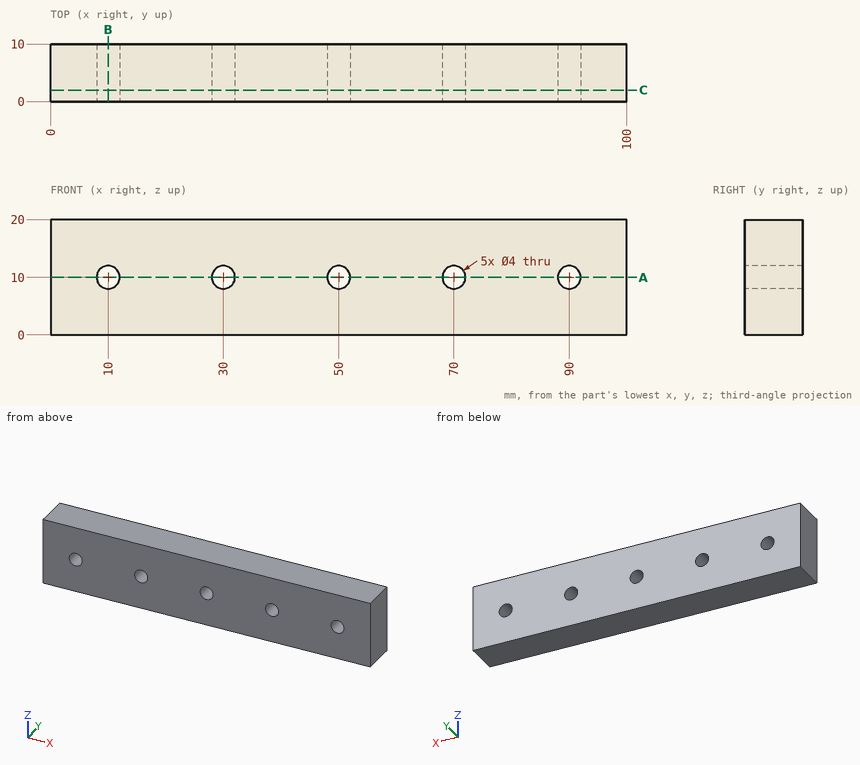
The drawing under review shows one solid part. Ordinate dimensions are in mm from its lowest x, y, z. Round coordinates to 2 decimals unless told otherwise and drop trailing zeros. Loops run counter-clockwise (first coordinate to the right, second up) from the corner with the lowest first, then second, coordinate; pieces in that order, holes last. Notation, with made-up numbers: (74, 9.5) - (129, 9.5) arc R22 cw to (129, 34.5) - close; hole circle Ø4 at (88, 21.5). An arc over 180 degrees is marked (long way). One line per item, written item: value. Start each with the question number.
1) To check wall thickness, follow L1, parallel to X at y = 2.5, z = 10; L2, parallel to Z at x = 30, y = 4.5; L3, parallel to X at y = 9.75, z = 8.5. State the ranges of each line that lie inside material, in increasing order. Write a range as from..to.
2) Insertion check: pin 1 Ø2.5 at (x, z) = (50, 10) entering from +Y; pin 2 Ø4.5 at (x, z) = (90, 10) entering from -Y. Each pin has a flat end and moves straight along its axis. Give the tip position at first contact, or say it passes through.
3) Consider section A-A on z = 10. Give the boundary of the cut face in (x, y), then the cut area to 3 significant figures.
4) Consider section C-C on y = 2. Give the boundary of the cut face in (x, z).
5) Consider section B-B on x = 10. Give the boundary of the cut face in (y, z), then the cut area to 3 significant figures.
Reported:
1. L1: x = 0..8, 12..28, 32..48, 52..68, 72..88, 92..100
1. L2: z = 0..8, 12..20
1. L3: x = 0..8.68, 11.32..28.68, 31.32..48.68, 51.32..68.68, 71.32..88.68, 91.32..100
2. pin 1: passes through
2. pin 2: stops at y = 0
3. outline: (0, 0) - (8, 0) - (8, 10) - (0, 10) - close; (12, 0) - (28, 0) - (28, 10) - (12, 10) - close; (32, 0) - (48, 0) - (48, 10) - (32, 10) - close; (52, 0) - (68, 0) - (68, 10) - (52, 10) - close; (72, 0) - (88, 0) - (88, 10) - (72, 10) - close; (92, 0) - (100, 0) - (100, 10) - (92, 10) - close
3. area: 800 mm^2
4. outline: (0, 0) - (100, 0) - (100, 20) - (0, 20) - close; hole circle Ø4 at (10, 10); hole circle Ø4 at (30, 10); hole circle Ø4 at (50, 10); hole circle Ø4 at (70, 10); hole circle Ø4 at (90, 10)
5. outline: (0, 0) - (10, 0) - (10, 8) - (0, 8) - close; (0, 12) - (10, 12) - (10, 20) - (0, 20) - close
5. area: 160 mm^2
